Part model, mm, in its own coordinate system. Face numbers are marked on the shaded views. A direction names the side the tool comes from. Round coordinates to 2 decimals unless told otherwise and drop trailing zeros. Loops run counter-clockwise (first coordinate to the right, second up) from the corner with the lowest first, then second, coordinate; pieces in that order, holes last. Notation, with made-up numbers: M 47,31.5 L 91,31.5 A18 ccw 91,50.5 Z; hole C -15,21 d5. An arc over 180 degrees is marked long. Put each result on its own line as item: value. Start each with the question number.
```python
from build123d import *

# Parameters (mm, degrees)
CROQUIS1_W                    = 40
CROQUIS1_H                    = 31.334822808
SALIENTE_EXTRUIR1_DEPTH       = 20
CROQUIS2_W                    = 5.048174606
CROQUIS2_H                    = 4.893641636
CORTAR_EXTRUIR1_DEPTH         = 41.340288801
TALADRO1_D                    = 6.35
TALADRO_DE_MARGEN_PARA_M221_D = 25.4
CROQUIS7_W                    = 20
CROQUIS7_H                    = 12.852705172
CROQUIS7_H_2                  = 13.588476
SALIENTE_EXTRUIR2_DEPTH       = 8
CROQUIS8_W                    = 48
CROQUIS8_H                    = 20
SALIENTE_EXTRUIR3_DEPTH       = 5
CROQUIS9_R                    = 3.175
CORTAR_EXTRUIR2_DEPTH         = 43
CROQUIS10_W                   = 48
CROQUIS10_H                   = 20
SALIENTE_EXTRUIR4_DEPTH       = 5
CORTAR_EXTRUIR3_START         = -48
CROQUIS11_R                   = 3.175
CORTAR_EXTRUIR3_DEPTH         = 48
CROQUIS12_R                   = 16.75
CORTAR_EXTRUIR4_DEPTH         = 48


with BuildPart() as part:
    # Croquis1 → Saliente-Extruir1 (new body)
    with BuildSketch(Plane(origin=(0, 0, 0), x_dir=(-1, 0, 0), z_dir=(0, 0, -1))):
        with Locations((11.334822808, 0)):
            Rectangle(CROQUIS1_W, CROQUIS1_H)
    extrude(amount=-SALIENTE_EXTRUIR1_DEPTH)

    # Croquis2 → Cortar-Extruir1 (cut, through all)
    with BuildSketch(Plane.XY.offset(20)):
        with Locations((6.141089889, 0.367885414)):
            Rectangle(CROQUIS2_W, CROQUIS2_H)
    extrude(amount=-CORTAR_EXTRUIR1_DEPTH, mode=Mode.SUBTRACT)

    # Taladro1 (through all)
    with Locations(Plane(origin=(0, 15.667411404, 0), x_dir=(1, 0, 0), z_dir=(0, 1, 0))):
        with Locations((-26.51855843, -10)):
            Hole(TALADRO1_D / 2)

    # Taladro de margen para M221 (through all)
    with Locations(Plane(origin=(0, 0, 0), x_dir=(-1, 0, 0), z_dir=(0, 0, -1))):
        with Locations((8.767354232, 0)):
            Hole(TALADRO_DE_MARGEN_PARA_M221_D / 2)

    # Croquis7 → Saliente-Extruir2 (add)
    with BuildSketch(Plane(origin=(8.665177192, 0, 0), x_dir=(0, 0, -1), z_dir=(1, 0, 0))):
        with Locations((-10, 9.241058818)):
            Rectangle(CROQUIS7_W, CROQUIS7_H)
        with Locations((-10, -8.873173404)):
            Rectangle(CROQUIS7_W, CROQUIS7_H_2)
    extrude(amount=SALIENTE_EXTRUIR2_DEPTH)

    # Croquis8 → Saliente-Extruir3 (add)
    with BuildSketch(Plane(origin=(0, 15.667411404, 0), x_dir=(1, 0, 0), z_dir=(0, 1, 0))):
        with Locations((-7.334822808, -10)):
            Rectangle(CROQUIS8_W, CROQUIS8_H)
    extrude(amount=SALIENTE_EXTRUIR3_DEPTH)

    # Croquis9 → Cortar-Extruir2 (cut)
    with BuildSketch(Plane.XZ.offset(15.667411404)):
        with Locations(Location((-26.51855843, 10, 0), (0, 0, 90))):
            Circle(CROQUIS9_R)
    extrude(amount=-CORTAR_EXTRUIR2_DEPTH, mode=Mode.SUBTRACT)

    # Croquis10 → Saliente-Extruir4 (add)
    with BuildSketch(Plane.XZ.offset(15.667411404)):
        with Locations((-7.334822808, 10)):
            Rectangle(CROQUIS10_W, CROQUIS10_H)
    extrude(amount=SALIENTE_EXTRUIR4_DEPTH)

    # Croquis11 → Cortar-Extruir3 (cut)
    with BuildSketch(Plane(origin=(0, 20.667411404, 0), x_dir=(1, 0, 0), z_dir=(0, 1, 0)).offset(CORTAR_EXTRUIR3_START)):
        with Locations(Location((-26.51855843, -10, 0), (0, 0, 90))):
            Circle(CROQUIS11_R)
    extrude(amount=CORTAR_EXTRUIR3_DEPTH, mode=Mode.SUBTRACT)

    # Croquis12 → Cortar-Extruir4 (cut)
    with BuildSketch(Plane.XY.offset(20)):
        with Locations((-4.925615177, 0)):
            Circle(CROQUIS12_R)
    extrude(amount=-CORTAR_EXTRUIR4_DEPTH, mode=Mode.SUBTRACT)


solid = part.part
```
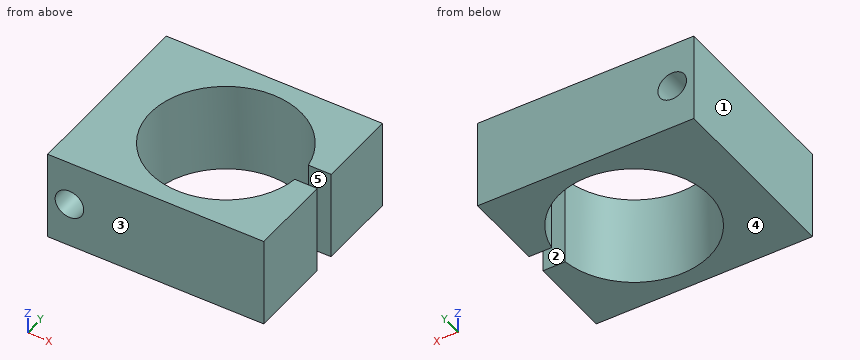
1. Mould opens along Y. For the marked faces 3, 4 and 5 say: released by +Y, released by -Y, zero draft, split by the parting line, or undercut.
2. Which spindle directions (+Z, -Z, +X, -X, +Y, -Y) get a long thin tool onto all of the face, cutting with end or side? Do the marked faces 1 and 2. Say none if no direction does.
3. Cut at C-C, the plane x = -7. Give the cut face in (y, z), and give its area (3 significant figures).
4. Cut at A-A, the plane z = 10. Give the cut face in (x, y).
5. Wall check: L1, parallel to X at y = -2.5, z = 11.75; L2, parallel to X at y = 9, z = 9.75; L3, parallel to X at y = 0, z = 10. Give the ranges that are in metal, low to high.
6. Cut at D-D, the plane z = 2.5. Give the cut face in (x, y), and give its area (3 significant figures).
7. Drop a flat-ended pin along its axis: pin 1 (4 mm diameter, centred on x = -25.5, z = 12.5, fed in from +Y). Give the stop position or say it passes through.
8. Cut at B-B, the plane y = -10.5. Give the cut face in (x, z) (3 decimals), and give its area (3 significant figures).
Results list:
1. face 3: released by -Y
1. face 4: zero draft
1. face 5: undercut
2. face 1: +Z, -Z, -X, +Y, -Y
2. face 2: +Z, -Z, +X
3. outline: M -20.67,0 L -16.62,0 L -16.62,20 L -20.67,20 Z; M 16.62,0 L 20.67,0 L 20.67,20 L 16.62,20 Z
3. area: 162 mm^2
4. outline: M -31.33,-20.67 L -29.69,-20.67 L -29.69,20.67 L -31.33,20.67 Z; M -23.34,-20.67 L 16.67,-20.67 L 16.67,-2.08 L 11.69,-2.08 A16.75 cw long 11.59,2.81 L 16.67,2.81 L 16.67,20.67 L -23.34,20.67 Z
5. L1: x = -31.33 to -29.17, -23.87 to -21.49, 11.64 to 16.67
5. L2: x = -31.33 to -29.68, -23.35 to -19.05, 9.2 to 16.67
5. L3: x = -31.33 to -29.69, -23.34 to -21.68
6. outline: M -31.33,-20.67 L 16.67,-20.67 L 16.67,-2.08 L 11.69,-2.08 A16.75 cw long 11.59,2.81 L 16.67,2.81 L 16.67,20.67 L -31.33,20.67 Z
6. area: 1,080 mm^2
7. pin 1: stops at y = 20.67
8. outline: M -31.335,0 L -17.976,0 L -17.976,20 L -31.335,20 Z; M 8.125,0 L 16.665,0 L 16.665,20 L 8.125,20 Z; hole C -26.519,10 d6.35
8. area: 406 mm^2
